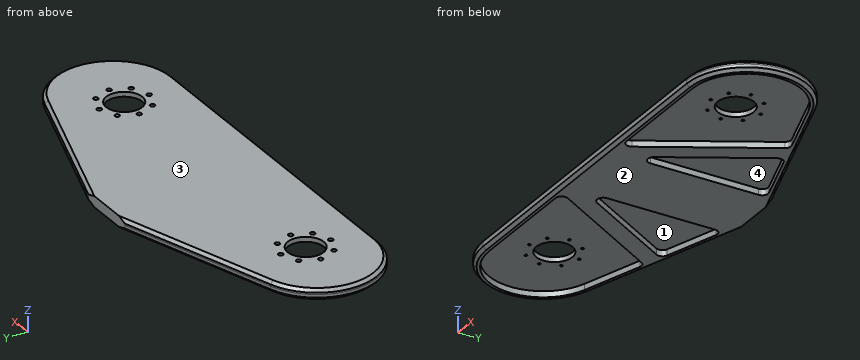
from build123d import *

# Parameters (mm, degrees)
SKETCH_1_R               = 30
EXTRUDE_1_DEPTH          = 8
FILLET_1_R               = 100
FILLET_3_R               = 100
EXTRUDE_2_DEPTH          = 10
FILLET_2_R               = 10
CHAMFER_1_SIZE           = 5
CUT_EXTRUDE_5_DEPTH      = 514.758413114
CUT_EXTRUDE_5_DEPTH_BACK = 514.758413114
SKETCH_8_R               = 2.25
SKETCH_9_R               = 4
CUT_EXTRUDE_6_DEPTH      = 4.4


with BuildPart() as part:
    # 草图1 → 凸台-拉伸1 (new body)
    with BuildSketch(Plane.XY):
        Polygon((0, 280), (861.751390409, 0), (0, 0), (-100, 0), (-961.751390409, 0), (-100, 280), align=None)
        with Locations((200, 100)):
            Circle(SKETCH_1_R, mode=Mode.SUBTRACT)
        with Locations(Location((-300, 100, 0), (0, 0, 180))):
            Circle(SKETCH_1_R, mode=Mode.SUBTRACT)
    extrude(amount=EXTRUDE_1_DEPTH)

    # 圆角1
    fillet_1_edges = [part.edges().sort_by_distance(p)[0] for p in [
        (861.751390409, 0, 4),
    ]]
    fillet(fillet_1_edges, radius=FILLET_1_R)

    # 圆角3
    fillet_3_edges = [part.edges().sort_by_distance(p)[0] for p in [
        (-961.751390409, 0, 4),
    ]]
    fillet(fillet_3_edges, radius=FILLET_3_R)

    # 草图2 → 凸台-拉伸2 (add)
    with BuildSketch(Plane.XY):
        with BuildLine():
            Line((0, 280), (-100, 280))
            Line((-100, 280), (-361.277938379, 195.10565163))
            ThreePointArc((-361.277938379, 195.10565163), (-429.145073001, 84.356553496), (-330.376238942, 0))
            Line((-330.376238942, 0), (230.376238942, 0))
            ThreePointArc((230.376238942, 0), (329.145073001, 84.356553496), (261.277938379, 195.10565163))
            Line((261.277938379, 195.10565163), (0, 280))
        make_face()
        Polygon((10, 266.236180795), (122.241374643, 229.766747442), (10, 35.358983849), align=None, mode=Mode.SUBTRACT)
        with BuildLine():
            Line((230.376238942, 10), (30, 10))
            Line((30, 10), (151.410485182, 220.289128906))
            Line((151.410485182, 220.289128906), (258.187768435, 185.595086467))
            ThreePointArc((258.187768435, 185.595086467), (319.268189595, 85.920898146), (230.376238942, 10))
        make_face(mode=Mode.SUBTRACT)
        Polygon((-110, 266.236180795), (-110, 35.358983849), (-222.241374643, 229.766747442), align=None, mode=Mode.SUBTRACT)
        with BuildLine():
            Line((-358.187768435, 185.595086467), (-251.410485182, 220.289128906))
            Line((-251.410485182, 220.289128906), (-130, 10))
            Line((-130, 10), (-330.376238942, 10))
            ThreePointArc((-330.376238942, 10), (-419.268189595, 85.920898146), (-358.187768435, 185.595086467))
        make_face(mode=Mode.SUBTRACT)
    extrude(amount=-EXTRUDE_2_DEPTH)

    # 圆角2
    fillet_2_edges = [part.edges().sort_by_distance(p)[0] for p in [
        (-110, 35.358983849, -5),
        (-110, 266.236180795, -5),
        (-130, 10, -5),
        (10, 266.236180795, -5),
        (10, 35.358983849, -5),
        (151.410485182, 220.289128906, -5),
        (30, 10, -5),
        (-251.410485182, 220.289128906, -5),
        (122.241374643, 229.766747442, -5),
        (-222.241374643, 229.766747442, -5),
    ]]
    fillet(fillet_2_edges, radius=FILLET_2_R)

    # 倒角1
    chamfer_1_edges = [part.edges().sort_by_distance(p)[0] for p in [
        (-230.63896919, 237.552825815, 8),
        (130.63896919, 237.552825815, 8),
        (329.145073001, 84.356553496, 8),
        (-50, 0, 8),
        (-429.145073001, 84.356553496, 8),
        (-230.63896919, 237.552825815, -10),
        (130.63896919, 237.552825815, -10),
        (329.145073001, 84.356553496, -10),
        (-50, 0, -10),
        (-429.145073001, 84.356553496, -10),
    ]]
    chamfer(chamfer_1_edges, length=CHAMFER_1_SIZE)

    # 草图8 → 切除-拉伸5 (cut, two sides: drawn at the far end of the back side and taken through both)
    with BuildSketch(Plane.XY.offset(8).offset(-CUT_EXTRUDE_5_DEPTH_BACK)):
        with Locations((200, 141.5)):
            Circle(SKETCH_8_R)
        with Locations((229.344931419, 129.344931419)):
            Circle(SKETCH_8_R)
        with Locations((241.5, 100)):
            Circle(SKETCH_8_R)
        with Locations((229.344931419, 70.655068581)):
            Circle(SKETCH_8_R)
        with Locations((200, 58.5)):
            Circle(SKETCH_8_R)
        with Locations((170.655068581, 70.655068581)):
            Circle(SKETCH_8_R)
        with Locations((158.5, 100)):
            Circle(SKETCH_8_R)
        with Locations((170.655068581, 129.344931419)):
            Circle(SKETCH_8_R)
        with Locations((-270.655068581, 129.344931419)):
            Circle(SKETCH_8_R)
        with Locations((-258.5, 100)):
            Circle(SKETCH_8_R)
        with Locations((-270.655068581, 70.655068581)):
            Circle(SKETCH_8_R)
        with Locations((-300, 58.5)):
            Circle(SKETCH_8_R)
        with Locations((-329.344931419, 70.655068581)):
            Circle(SKETCH_8_R)
        with Locations((-341.5, 100)):
            Circle(SKETCH_8_R)
        with Locations((-329.344931419, 129.344931419)):
            Circle(SKETCH_8_R)
        with Locations((-300, 141.5)):
            Circle(SKETCH_8_R)
    extrude(amount=CUT_EXTRUDE_5_DEPTH + CUT_EXTRUDE_5_DEPTH_BACK, mode=Mode.SUBTRACT)

    # 草图9 → 切除-拉伸6 (cut)
    with BuildSketch(Plane.XY.offset(8)):
        with Locations((-300, 141.5)):
            Circle(SKETCH_9_R)
        with Locations((-270.655068581, 129.344931419)):
            Circle(SKETCH_9_R)
        with Locations((-258.5, 100)):
            Circle(SKETCH_9_R)
        with Locations((-270.655068581, 70.655068581)):
            Circle(SKETCH_9_R)
        with Locations((-300, 58.5)):
            Circle(SKETCH_9_R)
        with Locations((-329.344931419, 70.655068581)):
            Circle(SKETCH_9_R)
        with Locations((-341.5, 100)):
            Circle(SKETCH_9_R)
        with Locations((-329.344931419, 129.344931419)):
            Circle(SKETCH_9_R)
        with Locations(Location((229.344931419, 129.344931419, 0), (0, 0, 180))):
            Circle(SKETCH_9_R)
        with Locations(Location((241.5, 100, 0), (0, 0, 180))):
            Circle(SKETCH_9_R)
        with Locations(Location((229.344931419, 70.655068581, 0), (0, 0, 180))):
            Circle(SKETCH_9_R)
        with Locations(Location((200, 58.5, 0), (0, 0, 180))):
            Circle(SKETCH_9_R)
        with Locations(Location((170.655068581, 70.655068581, 0), (0, 0, 180))):
            Circle(SKETCH_9_R)
        with Locations(Location((158.5, 100, 0), (0, 0, 180))):
            Circle(SKETCH_9_R)
        with Locations(Location((170.655068581, 129.344931419, 0), (0, 0, 180))):
            Circle(SKETCH_9_R)
        with Locations(Location((200, 141.5, 0), (0, 0, 180))):
            Circle(SKETCH_9_R)
    extrude(amount=-CUT_EXTRUDE_6_DEPTH, mode=Mode.SUBTRACT)


solid = part.part
Work out the finished part from the listing and answer in its coordinate system (mm). Face numbers are marked on the shaded views. A direction names the side the tool comes from. Give positions to 0.01 mm unless a question says otherwise; leave off trailing zeros. Write each loop counter-clockwise with the first axis right and the second up, starting at its lowest first coordinate (ties: lowest second). Pieces come first, ordered by that corner, then holes.
Q1. A tool of negligible diameter and unlimited length cuts with its end or side. For the marked faces 1 and 2, from which of +Z, -Z, +X, -X, +Y, -Y can it reach the whole face along a straight path? Write none if from no direction.
Answer:
face 1: -Z
face 2: -Z, +X, -X, +Y, -Y
Q2. Straight lines are drawn through the part: L1, parallel to Y at x = 200, z = 1.05; L2, parallel to X at y = 170, z = -8.25; L3, parallel to X at y = 141.5, z = 1.95. For each, find the intervals that lie inside material, in ascending order.
Answer:
L1: y = 0 to 56.25, 60.75 to 70, 130 to 139.25, 143.75 to 215.02
L2: x = -397.16 to -386.94, -222.38 to -187.74, -110 to 10, 87.74 to 122.38, 286.94 to 297.16
L3: x = -421.36 to -302.25, -297.75 to 197.75, 202.25 to 321.36
Q3. Given pin 1 (6 mm diameter, centred on x = 229.34, y = 129.34, fed in from -Z); pin 2 (3 mm diameter, centred on y = 185.5, z = -6.5, fed in from -X); pin 3 (8 mm diameter, centred on y = 116, z = -7.5, fed in from +X), each flat-ended and moving along its own axis, determine where each tip first touches the part or whether it passes through.
Answer:
pin 1: stops at z = 0
pin 2: stops at x = -383.14
pin 3: stops at x = 329.54
Q4. The part is cut by section B-B on x = -182.5. Give the vertices of the cut face in (y, z), and give its area (3 significant figures).
Answer:
outline: (0, -5) - (5, -10) - (10, -10) - (10, 0) - (100.93, 0) - (100.93, -10) - (160.93, -10) - (160.93, 0) - (242.68, 0) - (242.68, -10) - (247.94, -10) - (253.19, -5) - (253.19, 3) - (247.94, 8) - (5, 8) - (0, 3) - close
area: 2,780 mm2
Q5. The part is cut by section A-A on x = 187.5. Give the vertices of the cut face in (y, z), and give its area (3 significant figures).
Answer:
outline: (0, -5) - (5, -10) - (10, -10) - (10, 0) - (72.73, 0) - (72.73, 8) - (5, 8) - (0, 3) - close; (127.27, 0) - (208.56, 0) - (208.56, -10) - (213.82, -10) - (219.08, -5) - (219.08, 3) - (213.82, 8) - (127.27, 8) - close
area: 1,470 mm2
Q6. For a pull along X with two mould halves and no side action, classify the marked faces 3 and 4 as released by +X, released by -X, zero draft, split by the parting line, or undercut.
Answer:
face 3: zero draft
face 4: undercut
